The model under review builds one solid part; all positions refer to its coordinate system, in mm. Face numbers are marked on the shaded views. A direction names the side the tool comes from. Give positions to 0.01 mm unless a question says otherwise; leave off trailing zeros. Write each loop counter-clockwise with the first axis right and the second up, starting at its lowest first coordinate (ties: lowest second). Pieces come first, ordered by that corner, then holes.
from build123d import *

# Parameters (mm, degrees)
F0_W     = 6.35
F0_H     = 42.3414773719
F1_DEPTH = 3.81
F3_ANGLE = 180
F4_T     = -1.27
F7_DEPTH = 25.4


# Not quite as in the source:
# - a feature names something its author has since deleted; it is built from what else it names


with BuildPart() as f1:
    # F0 (on Top) → F1 (new body)
    with BuildSketch(Plane.XY):
        Polygon((6.35, -30.48), (6.35, -35.56), (9.1898063314, -33.02), align=None)
        Polygon((6.35, -35.56), (6.35, -40.64), (9.1898063314, -38.1), align=None)
        Polygon((6.35, -25.4), (6.35, -30.48), (9.1898063314, -27.94), align=None)
        Polygon((6.35, -20.32), (6.35, -25.4), (9.1898063314, -22.86), align=None)
        Polygon((9.1898063314, -17.78), (6.35, -15.24), (6.35, -20.32), align=None)
        Polygon((9.1898063314, -12.7), (6.35, -10.16), (6.35, -15.24), align=None)
        Polygon((9.1898063314, -7.62), (6.35, -5.08), (6.35, -10.16), align=None)
        Polygon((9.1898063314, -2.54), (6.35, 0), (6.35, -5.08), align=None)
        Polygon((6.35, 0), (0, 0), (0, -42.3414773719), (6.35, -40.64), (6.35, -35.56), (6.35, -30.48), (6.35, -25.4), (6.35, -20.32), (6.35, -15.24), (6.35, -10.16), (6.35, -5.08), align=None)
        with Locations((-3.175, -21.170738686)):
            Rectangle(F0_W, F0_H)
    extrude(amount=F1_DEPTH)


with BuildPart() as f3:
    # F2 (on face) → F3 (revolve)
    with BuildSketch(Plane.XY.offset(3.81)):
        with BuildLine():
            ThreePointArc((10.16, 5.08), (5.6796126628, 1.3407746743), (0, 0))
            Line((0, 0), (6.35, 0))
            Line((6.35, 0), (10.16, 5.08))
        make_face()
        with BuildLine():
            Line((0, 25.4), (0, 0))
            ThreePointArc((0, 0), (5.6796126628, 1.3407746743), (10.16, 5.08))
            ThreePointArc((10.16, 5.08), (11.3592253257, 18.3796126628), (0, 25.4))
        make_face()
    revolve(axis=Axis((0, 12.7, 3.81), (0, 1, 0)), revolution_arc=F3_ANGLE)

    # F4
    f4_openings = [f3.faces().sort_by_distance(p)[0] for p in [
        (0, 12.436594, 3.81),
    ]]
    offset(amount=F4_T, openings=f4_openings)


with BuildPart() as f1_1:
    add(f1.part)

    # F5: union F3
    add(f3.part)

    # F6 (on face) → F7 (cut)
    with BuildSketch(Plane.XY.offset(3.81)):
        with BuildLine():
            Line((8.9097454996, 19.8597021678), (9.4470019608, 21.1878827721))
            ThreePointArc((9.4470019608, 21.1878827721), (5.1717448117, 24.299269615), (0, 25.4))
            ThreePointArc((0, 25.4), (-1.5546529222, 25.304485483), (-3.0859212896, 25.0193786286))
            Line((-3.0859212896, 25.0193786286), (-2.5834265714, 23.8342178508))
            ThreePointArc((-2.5834265714, 23.8342178508), (-1.3001519074, 24.0558137101), (0, 24.13))
            ThreePointArc((0, 24.13), (1.2447495309, 24.0620200055), (2.4746927509, 23.8588886449))
            Line((2.4746927509, 23.8588886449), (2.9447663441, 25.0209828664))
            Line((2.9447663441, 25.0209828664), (3.5641672216, 23.5600926339))
            ThreePointArc((3.5641672216, 23.5600926339), (6.5056012054, 22.0979813234), (8.9097454996, 19.8597021678))
        make_face()
        with BuildLine():
            Line((7.0658245088, 15.3012458764), (8.9097454996, 19.8597021678))
            ThreePointArc((8.9097454996, 19.8597021678), (6.5056012054, 22.0979813234), (3.5641672216, 23.5600926339))
            Line((3.5641672216, 23.5600926339), (7.0658245088, 15.3012458764))
        make_face()
        with BuildLine():
            ThreePointArc((2.4746927509, 23.8588886449), (3.0231237497, 23.7229588947), (3.5641672216, 23.5600926339))
            Line((3.5641672216, 23.5600926339), (2.9447663441, 25.0209828664))
            Line((2.9447663441, 25.0209828664), (2.4746927509, 23.8588886449))
        make_face()
        with BuildLine():
            Line((-2.5834265714, 23.8342178508), (-3.0859212896, 25.0193786286))
            ThreePointArc((-3.0859212896, 25.0193786286), (-3.1028243507, 25.0151321978), (-3.1197215685, 25.0108625748))
            Line((-3.1197215685, 25.0108625748), (-3.7290136249, 23.5045988998))
            ThreePointArc((-3.7290136249, 23.5045988998), (-3.1605201267, 23.6843530774), (-2.5834265714, 23.8342178508))
        make_face()
        with BuildLine():
            Line((0, 17.7410675473), (2.4746927509, 23.8588886449))
            ThreePointArc((2.4746927509, 23.8588886449), (1.2447495309, 24.0620200055), (0, 24.13))
            ThreePointArc((0, 24.13), (-1.3001519074, 24.0558137101), (-2.5834265714, 23.8342178508))
            Line((-2.5834265714, 23.8342178508), (0, 17.7410675473))
        make_face()
        with BuildLine():
            Line((-3.7290136249, 23.5045988998), (-3.1197215685, 25.0108625748))
            ThreePointArc((-3.1197215685, 25.0108625748), (-6.6419627447, 23.5247092754), (-9.562361361, 21.0577057379))
            Line((-9.562361361, 21.0577057379), (-9.0040057437, 19.7407940296))
            ThreePointArc((-9.0040057437, 19.7407940296), (-6.6388253732, 22.0043483202), (-3.7290136249, 23.5045988998))
        make_face()
        with BuildLine():
            Line((-7.0836272172, 15.211478147), (-3.7290136249, 23.5045988998))
            ThreePointArc((-3.7290136249, 23.5045988998), (-6.6388253732, 22.0043483202), (-9.0040057437, 19.7407940296))
            Line((-9.0040057437, 19.7407940296), (-7.0836272172, 15.211478147))
        make_face()
    extrude(amount=-F7_DEPTH, mode=Mode.SUBTRACT)


solid = f1_1.part
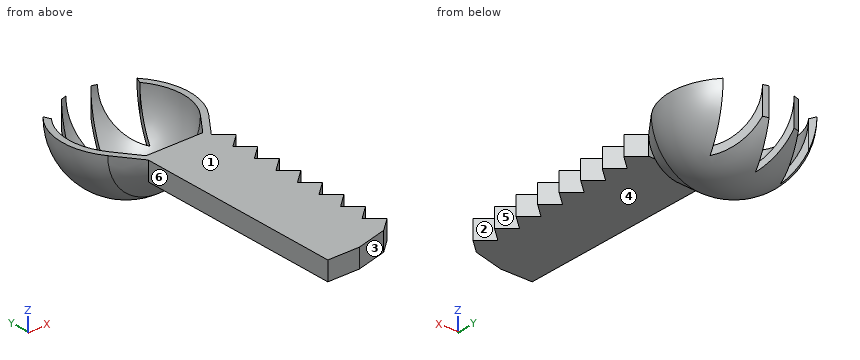
1) Insertion check: pin 1 (4 mm diameter, centred on x = 5, z = -4, fed in from +Y); pin 2 (12 mm diameter, centred on x = 6, y = -3, fed in from -Z); pin 3 (0.6 mm diameter, centred on x = 5.5, z = 2.5, fed in from +Y). Each pin has a flat end and moves straight along its axis. Give the tip position at first contact, or say it passes through.
2) Consider section B-B, the plane y = -18.5. Give the boundary of the cut face in (x, z).
3) To check wall thickness, follow probe 1 along X at (y, z) = (16, -5); probe 2 along Z at (x, y) = (-4, -21); probe 3 along Y at (x, z) = (9.25, 0). State the ranges of each line that lie inside material, in increasing order.
4) Tool access review of the marked faces 4, 5 and 6: name each direction out of +Z, -Z, +X, -X, +Y, -Y from which nothing blocks a thin tool from reaching the whole face with its end or side.
5) Consider section A-A, the plane z = -1. State how many separate pieces and enclosed holes the cut face has, then the cut area to 3 significant figures.
6) The part is to be moulded in two halves that separate along Y. For the marked faces 1, 2 and 3, say which applies: +Y half, -Y half, draft (parallel to the pull), parting line (faces both ways), or undercut.
Answer block:
1. pin 1: stops at y = 23.1
1. pin 2: stops at z = -3.61
1. pin 3: stops at y = 1.59
2. outline: (-6.35, 0) - (8.38, 0) - (8.38, 3.81) - (-6.35, 3.81) - close
3. probe 1: x = -8.53 to -7.42, -6.76 to -6.49, 6.49 to 6.77, 7.35 to 8.53
3. probe 2: z = 0 to 3.81
3. probe 3: y = 4.87 to 7.17, 18.23 to 20.52
4. face 4: -Z, +X, -X, -Y
4. face 5: +Z, -Z, +X
4. face 6: +Z, -Z, -X, -Y
5. separate pieces: 3
5. enclosed holes: 0
5. area: 74.6 mm2
6. face 1: draft
6. face 2: undercut
6. face 3: -Y half
